Read the model definition and answer for the solid it produces. Units are mm, in the model's axes. Give positions to 0.01 mm unless a question says otherwise; leave off trailing zeros. Loops run counter-clockwise (first coordinate to the right, second up) from the corner with the lowest first, then second, coordinate; pieces in that order, holes last. Notation, with made-up numbers: (-21, -29) - (8, -29) arc R14 ccw to (8, -6) - close; hole circle Ø9 at (68.5, 53). An arc over 180 degrees is marked (long way). Put each result on its own line as item: value. Start each with the question number.
1. Consider L1, parallel to X at y = 8, z = 0.4; L2, parallel to Y at x = -19.5, z = 0.3; L3, parallel to X at y = -4.5, z = 0.95. Determine where each line is inside the solid, lowest interval first. Write a range as from..to.
2. A cutting plane is placed at A-A, the plane z = 0.85. Determine the outline of the cut face in (x, y), plus the area to 3 significant figures.
3. A cutting plane is placed at C-C, the plane x = -21. Determine the outline of the cut face in (y, z), plus the area to 3 significant figures.
4. A cutting plane is placed at B-B, the plane y = -20.5. Determine the outline of the cut face in (x, z).
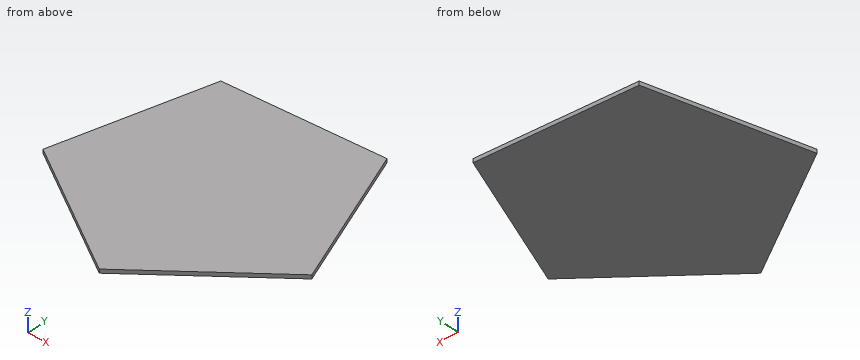
```python
from build123d import *

# Parameters (mm, degrees)
F1_DEPTH = 1


with BuildPart() as f1:
    # F0 (on Top) → F1 (new body)
    with BuildSketch(Plane.XY):
        Polygon((19.1758844015, 25.326287722), (-22.4985656812, 22.4124055891), (-32.6054123978, -18.1227908238), (2.822662895, -40.2610378147), (34.8252642985, -13.4080304936), align=None)
        Polygon((-31.7215240873, -17.8355981024), (-21.9522926631, 21.6605252833), (18.6296113834, 24.5744074162), (33.941375988, -13.1208377722), (2.822662895, -39.3316626458), align=None, mode=Mode.SUBTRACT)
        Polygon((18.6296113834, 24.5744074162), (-21.9522926631, 21.6605252833), (-31.7215240873, -17.8355981024), (2.822662895, -39.3316626458), (33.941375988, -13.1208377722), align=None)
    extrude(amount=F1_DEPTH)


solid = f1.part
```
Return value:
1. L1: x = -26.09..26.18
1. L2: y = -26.31..22.62
1. L3: x = -29.21..31.23
2. outline: (-32.61, -18.12) - (2.82, -40.26) - (34.83, -13.41) - (19.18, 25.33) - (-22.5, 22.41) - close
2. area: 3,000 mm2
3. outline: (-25.37, 0) - (22.52, 0) - (22.52, 1) - (-25.37, 1) - close
3. area: 47.9 mm2
4. outline: (-28.8, 0) - (26.37, 0) - (26.37, 1) - (-28.8, 1) - close
